CAD build for the part. Positions are in the model's coordinates, mm. Give positions to 0.01 mm unless a question says otherwise; leave off trailing zeros. Order: outer loops, then holes, each group sorted by start corner. A loop starts at its lowest first (then second) coordinate and runs counter-clockwise, first axis right, second up.
Item 1: Band-saw the part on D-D on z = 42.5. Give the cut face in (x, y) (3 decimals), plus the area to 3 significant figures.
Item 2: Band-saw the part on B-B on y = -0.35. Give the cut face in (x, z) (1 decimal), plus the area to 3 significant figures.
Item 3: Band-saw the part on A-A on z = 0. Give the cut face in (x, y) (3 decimals).
Item 4: Band-saw the part on C-C on x = 0. Give the cut face in (y, z) (3 decimals).
Item 5: Wall check: L1, parallel to Z at x = -0.5, y = -0.55; L2, parallel to X at y = -0.1, z = 18.5; L3, parallel to Z at x = 16, y = 0.25. Give the ranges that are in metal, low to high.
Item 6: Flat gauge pins, fed straight in: P1, Ø2, axis at x = -29.5, z = -19, coming from the -Y side; P2, Ø0.7, axis at y = -0.5, z = -35, coming from the -X side. Where does each tip first touch, or does it go through?
```python
from build123d import *

# Parameters (mm, degrees)
SKETCH1_R                = 54
SKETCH1_R_2              = 37.6
BOSS_EXTRUDE1_DEPTH      = 0.725
BOSS_EXTRUDE2_DEPTH      = 0.725
FILLET1_R                = 0.8
CIRPATTERN1_COUNT        = 3
FILLET1_OF_CIRPATTERN1_R = 0.8


with BuildPart() as part:
    # Sketch1 → Boss-Extrude1 (new, symmetric)
    with BuildSketch(Plane(origin=(0, 0, 0), x_dir=(1, 0, 0), z_dir=(0, 1, 0))):
        with Locations(Location((0, 0, 0), (0, 0, 270))):
            Circle(SKETCH1_R)
        with Locations(Location((0, 0, 0), (0, 0, 270))):
            Circle(SKETCH1_R_2, mode=Mode.SUBTRACT)
    extrude(amount=BOSS_EXTRUDE1_DEPTH, both=True)

    # Sketch2 → Boss-Extrude2 (add, symmetric)
    with BuildSketch(Plane(origin=(0, 0, 0), x_dir=(1, 0, 0), z_dir=(0, 1, 0))):
        with BuildLine():
            Line((-5.875, 32.6), (5.875, 32.6))
            Line((5.875, 32.6), (5.875, 37.138179479))
            ThreePointArc((5.875, 37.138179479), (0, 37.6), (-5.875, 37.138179479))
            Line((-5.875, 37.138179479), (-5.875, 32.6))
        make_face()
    boss_extrude2 = extrude(amount=BOSS_EXTRUDE2_DEPTH, both=True)

    # Fillet1
    fillet1_edges = [part.edges().sort_by_distance(p)[0] for p in [
        (-5.875, 0, -37.138179479),
        (5.875, 0, -37.138179479),
    ]]
    fillet(fillet1_edges, radius=FILLET1_R)

    # CirPattern1: Boss-Extrude2 ×3 about axis
    cirpattern1_axis = Axis((0, 0, 0), (0, 1, 0))
    for i in range(1, CIRPATTERN1_COUNT):
        add(boss_extrude2.rotate(cirpattern1_axis, i * 360 / CIRPATTERN1_COUNT))

    # Fillet1 of CirPattern1
    fillet1_of_cirpattern1_edges = [part.edges().sort_by_distance(p)[0] for p in [
        (-29.225106879, 0, 23.656988987),
        (-35.100106879, 0, 13.481190492),
        (35.100106879, 0, 13.481190492),
        (29.225106879, 0, 23.656988987),
    ]]
    fillet(fillet1_of_cirpattern1_edges, radius=FILLET1_OF_CIRPATTERN1_R)


solid = part.part
```
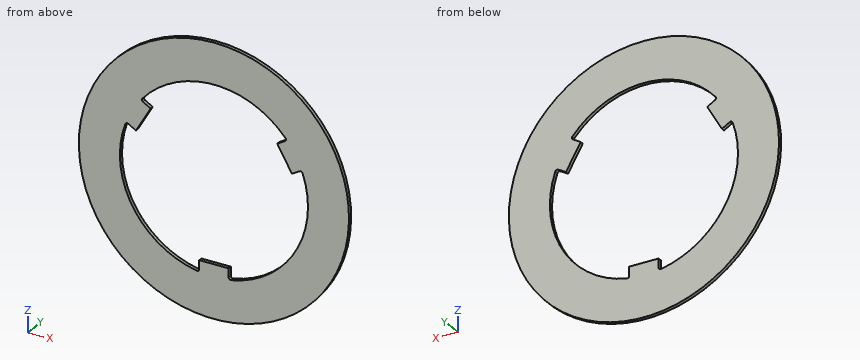
The answers:
1. outline: (-33.313, -0.725) - (33.313, -0.725) - (33.313, 0.725) - (-33.313, 0.725) - close
1. area: 96.6 mm2
2. outline: circle Ø108 at (0, 0); hole (-35.4, 12.6) arc R37.6 ccw to (-6.8, -37) arc R0.8 ccw to (-5.9, -36.2) - (-5.9, -32.6) - (5.9, -32.6) - (5.9, -36.2) arc R0.8 ccw to (6.8, -37) arc R37.6 ccw to (35.4, 12.6) arc R0.8 ccw to (34.3, 13) - (31.2, 11.2) - (25.3, 21.4) - (28.4, 23.2) arc R0.8 ccw to (28.6, 24.4) arc R37.6 ccw to (-28.6, 24.4) arc R0.8 ccw to (-28.4, 23.2) - (-25.3, 21.4) - (-31.2, 11.2) - (-34.3, 13) arc R0.8 ccw to start
2. area: 4,890 mm2
3. outline: (-54, -0.725) - (-37.6, -0.725) - (-37.6, 0.725) - (-54, 0.725) - close; (37.6, -0.725) - (54, -0.725) - (54, 0.725) - (37.6, 0.725) - close
4. outline: (-0.725, -54) - (0.725, -54) - (0.725, -32.6) - (-0.725, -32.6) - close; (-0.725, 37.6) - (0.725, 37.6) - (0.725, 54) - (-0.725, 54) - close
5. L1: z = -54 to -32.6, 37.6 to 54
5. L2: x = -50.73 to -26.96, 26.96 to 50.73
5. L3: z = -51.58 to -34.03, 34.03 to 51.58
6. P1: passes through
6. P2: stops at x = -41.42
